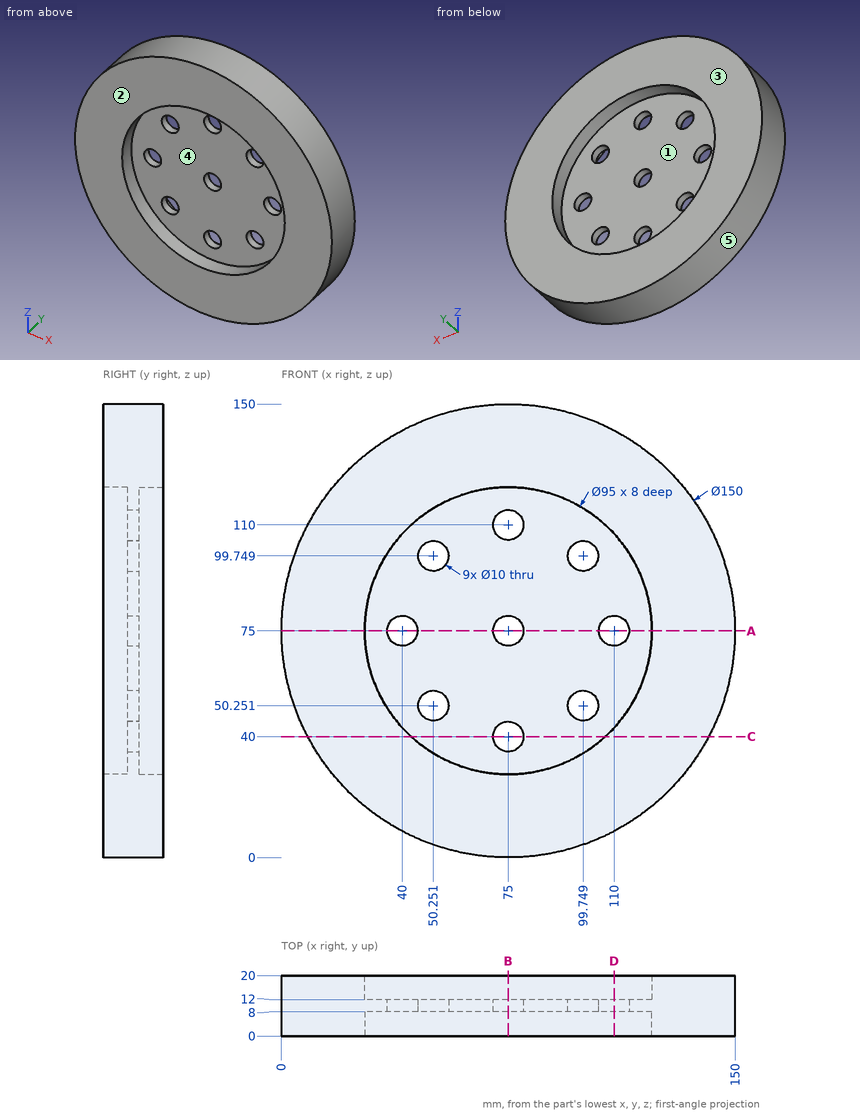
Answer from the drawing. Dimensions are ordinates in mm from the lowest x, y and z of the part. A direction names the side the tool comes from. Coordinates: 2 decimals unless noted, no trailing zeros. Write each loop counter-clockwise with the first axis right and the second up, starting at its lowest first coordinate (ties: lowest second). Pieces come first, ordered by that corner, then holes. Notation, with made-up numbers: (38.25, 56) - (58.25, 56) arc R11 ccw to (58.25, 70) - close; hole circle Ø5 at (-8.5, 70.5). An arc over 180 degrees is marked (long way). Return JSON: item names as keys, results as strings. Group by question number.
Q1. The part is cut by section C-C on z = 40. Write down the section's boundary in (x, y).
Q2. Flat-ended cylindrical pins translate along their axes: pin 1 Ø11.5 at (x, z) = (99.75, 99.75) entering from +Y; pin 2 Ø6 at (y, z) = (12, 62.5) entering from -X; pin 3 Ø1.5 at (y, z) = (13, 111.5) entering from +X. Find the tip coordinate at first contact, or state that the pin passes through.
Q3. The part is cut by section A-A on z = 75. Write down the section's boundary in (x, y), and give its area (3 significant figures).
Q4. For a pull along X with two mould halves and no side action, classify the marked faces 3, 4 and 5 as +X half, -X half, draft (parallel to the pull), parting line (faces both ways), or undercut.
Q5. The part is cut by section B-B on x = 75. Write down the section's boundary in (y, z), and give its area (3 significant figures).
Q6. Which of the six approach directions +Z, -Z, +X, -X, +Y, -Y give full straight-line access (tool end or side, diameter ignored) to the marked faces 1 and 2?
Q7. The part is cut by section D-D on x = 110. Write down the section's boundary in (y, z).
Q8. Find the intervals of material crossed by line 1 along X through (y, z) = (10.5, 75); line 2 along Z through (x, y) = (75, 15), in increasing order. Write a range as [from, to].
Evaluation:
{
 "1": {"outline": "(8.67, 0) - (42.89, 0) - (42.89, 8) - (70, 8) - (70, 12) - (42.89, 12) - (42.89, 20) - (8.67, 20) - close; (80, 8) - (107.11, 8) - (107.11, 0) - (141.33, 0) - (141.33, 20) - (107.11, 20) - (107.11, 12) - (80, 12) - close"},
 "2": {"pin 1": "stops at y = 12", "pin 2": "stops at x = 0.6", "pin 3": "stops at x = 140.93"},
 "3": {"outline": "(0, 0) - (27.5, 0) - (27.5, 8) - (35, 8) - (35, 12) - (27.5, 12) - (27.5, 20) - (0, 20) - close; (45, 8) - (70, 8) - (70, 12) - (45, 12) - close; (80, 8) - (105, 8) - (105, 12) - (80, 12) - close; (115, 8) - (122.5, 8) - (122.5, 0) - (150, 0) - (150, 20) - (122.5, 20) - (122.5, 12) - (115, 12) - close", "area": "1,360 mm2"},
 "4": {"face 3": "draft", "face 4": "undercut", "face 5": "parting line"},
 "5": {"outline": "(0, 0) - (20, 0) - (20, 27.5) - (12, 27.5) - (12, 35) - (8, 35) - (8, 27.5) - (0, 27.5) - close; (0, 122.5) - (8, 122.5) - (8, 115) - (12, 115) - (12, 122.5) - (20, 122.5) - (20, 150) - (0, 150) - close; (8, 45) - (12, 45) - (12, 70) - (8, 70) - close; (8, 80) - (12, 80) - (12, 105) - (8, 105) - close", "area": "1,360 mm2"},
 "6": {"face 1": "+Y", "face 2": "+Z, -Z, +X, -X, -Y"},
 "7": {"outline": "(0, 8.67) - (20, 8.67) - (20, 42.89) - (12, 42.89) - (12, 70) - (8, 70) - (8, 42.89) - (0, 42.89) - close; (0, 107.11) - (8, 107.11) - (8, 80) - (12, 80) - (12, 107.11) - (20, 107.11) - (20, 141.33) - (0, 141.33) - close"},
 "8": {"line 1": "x = [0, 35], [45, 70], [80, 105], [115, 150]", "line 2": "z = [0, 27.5], [122.5, 150]"}
}
